Geometry check sheet. Reference: the model listing, model coordinates, mm. A direction names the side the tool comes from. Give positions to 0.01 mm unless a question says otherwise; leave off trailing zeros. Order: outer loops, then holes, each group sorted by start corner. A loop starts at its lowest first (then second) coordinate and runs counter-clockwise, first axis right, second up. Notation, with made-up numbers: M 82.25,8 L 117.25,8 A26 ccw 117.25,38 Z; hole C -2,28.5 d11. An arc over 180 degrees is marked long. Put each result on its own line as item: value. Start each with the question number.
Q1. Go/stop test with flat-tipped pins: pin 1 (2 mm diameter, centred on x = 4.5, z = 1, fed in from +Y); pin 2 (1 mm diameter, centred on x = 13, z = -2.5, fed in from +Y); pin 3 (0.6 mm diameter, centred on y = 1.5, z = -2, fed in from -X); pin 4 (4 mm diameter, centred on x = 7, z = -3, fed in from +Y). Record where each tip stops, or that it passes through.
Q2. Mould release check, pull along Z, two halves, no side actions. Record for faces 1 (the flat face through (0, -3.1, 0.1)), 2 (the cylindrical face through (12, 0, 3)), 3 (the flat face through (1.233, 2.219, -1.257)), 4 (the flat face through (1, 0, -2.55)): +Z half, -Z half, draft (parallel to the pull), parting line (faces both ways), or undercut.
Q3. Material ranges on L1, parallel to X at y = 4.25, z = -1; L2, parallel to X at y = 1.5, z = -0.75; L3, parallel to Y at x = 14.75, z = 0, recorded low to high.
Q4. Section check A-A on x = 17.25. Record the cut outline in (y, z).
Q5. Access from +Z, -Z, +X, -X, +Y, -Y to the whole of each face (thin tool, end or side, straight path). Record for faces 5 (the flat face through (6, -1.1, -3.3)), 6 (the flat face through (1.23, 2.2, 1.29)), 7 (the cylindrical face through (3.11, 1.532, 4.864)).
```python
from build123d import *

# Parameters (mm, degrees)
ESBO_O1_W                = 6
ESBO_O1_H                = 5.1
ESBO_O2_R                = 3
RESSALTO_EXTRUS_O1_DEPTH = 12
CORTE_EXTRUS_O1_DEPTH    = 2.5
CHANFRO1_SIZE            = 0.3
FILETE1_R                = 0.2


with BuildPart() as part:
    # Esboço1 → Revolução1 (revolve)
    with BuildSketch(Plane(origin=(0, 0, 0), x_dir=(-1, 0, 0), z_dir=(0, 0, -1)), mode=Mode.PRIVATE) as revolu_o1_sk:
        with Locations((-3, 2.55)):
            Rectangle(ESBO_O1_W, ESBO_O1_H)
    revolve(revolu_o1_sk.sketch.rotate(Axis((6, 0, 0), (-1, 0, 0)), 270), axis=Axis((6, 0, 0), (-1, 0, 0)))

    # Esboço2 → Ressalto-extrusão1 (add)
    with BuildSketch(Plane(origin=(6, 0, 0), x_dir=(0, 0, -1), z_dir=(1, 0, 0))):
        Circle(ESBO_O2_R)
    extrude(amount=RESSALTO_EXTRUS_O1_DEPTH)

    # Esboço3 → Corte-extrusão1 (cut)
    with BuildSketch(Plane.ZY):
        Polygon((0, 2.944486373), (-2.55, 1.472243186), (-2.55, -1.472243186), (0, -2.944486373), (2.55, -1.472243186), (2.55, 1.472243186), align=None)
    extrude(amount=-CORTE_EXTRUS_O1_DEPTH, mode=Mode.SUBTRACT)

    # Esboço4 → Corte-Revolução1 (revolve, cut)
    with BuildSketch(Plane.XY, mode=Mode.PRIVATE) as corte_revolu_o1_sk:
        Polygon((2.5, 2.55), (2.5, 0), (3.972243186, 0), align=None)
    revolve(corte_revolu_o1_sk.sketch.rotate(Axis((2.5, 0, 0), (1, 0, 0)), 180), axis=Axis((2.5, 0, 0), (1, 0, 0)), mode=Mode.SUBTRACT)

    # Chanfro1
    chanfro1_edges = [part.edges().sort_by_distance(p)[0] for p in [
        (18, 0, 3),
        (0, 0, -5.1),
    ]]
    chamfer(chanfro1_edges, length=CHANFRO1_SIZE)

    # Filete1
    filete1_edges = [part.edges().sort_by_distance(p)[0] for p in [
        (6, 0, 3),
    ]]
    fillet(filete1_edges, radius=FILETE1_R)

    # Sketch1 → Cut-Revolve1 (revolve, cut)
    with BuildSketch(Plane(origin=(0, 0, 0), x_dir=(1, 0, 0), z_dir=(0, 1, 0)), mode=Mode.PRIVATE) as cut_revolve1_sk:
        Polygon((0, 2.945), (1.700296543, 0), (0, 0), align=None)
    revolve(cut_revolve1_sk.sketch.rotate(Axis((1.700296543, 0, 0), (1, 0, 0)), 180), axis=Axis((1.700296543, 0, 0), (1, 0, 0)), mode=Mode.SUBTRACT)


solid = part.part
```
Results found:
1. pin 1: stops at y = 5.1
1. pin 2: stops at y = 2.24
1. pin 3: stops at x = 0.08
1. pin 4: stops at y = 4.94
2. face 1: draft
2. face 2: parting line
2. face 3: undercut
2. face 4: undercut
3. L1: x = 0 to 6
3. L2: x = 3 to 18
3. L3: y = -3 to 3
4. outline: C 0,0 d6
5. face 5: +X
5. face 6: -X
5. face 7: +X, -X
